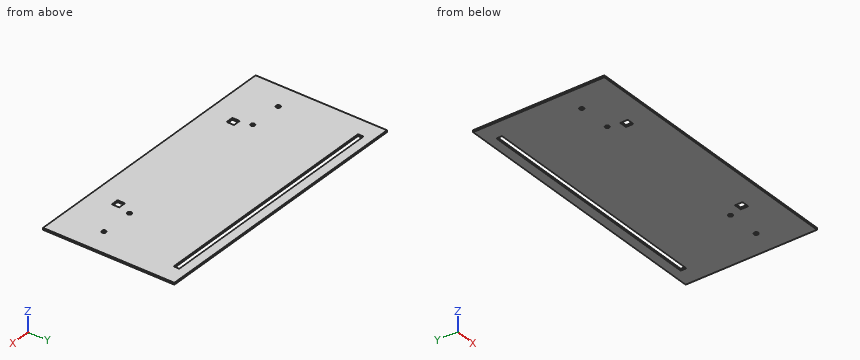
```python
from build123d import *

# Parameters (mm, degrees)
SK_PANEL_W            = 300
SK_PANEL_H            = 141.5
EX_PANEL_DEPTH        = 2
SK_LIGHTSLOT_W        = 260
SK_LIGHTSLOT_H        = 6
CUT_LIGHTSLOT_DEPTH   = 2
SK_CLIFFBOLTS_R       = 2.25
CUT_CLIFFBOLTS_DEPTH  = 2
SK_CLIFFCABLES_W      = 8
SK_CLIFFCABLES_H      = 8
CUT_CLIFFCABLES_DEPTH = 2


with BuildPart() as part:
    # SK_Panel → EX_Panel (new body)
    with BuildSketch(Plane.XY):
        with Locations((0, 70.75)):
            Rectangle(SK_PANEL_W, SK_PANEL_H)
    extrude(amount=EX_PANEL_DEPTH)

    # SK_LightSlot → CUT_LightSlot (cut)
    with BuildSketch(Plane.XY):
        with Locations((0, 128.5)):
            Rectangle(SK_LIGHTSLOT_W, SK_LIGHTSLOT_H)
    extrude(amount=CUT_LIGHTSLOT_DEPTH, mode=Mode.SUBTRACT)

    # SK_CliffBolts → CUT_CliffBolts (cut)
    with BuildSketch(Plane.XY):
        with Locations((123, 45)):
            Circle(SK_CLIFFBOLTS_R)
        with Locations((87, 45)):
            Circle(SK_CLIFFBOLTS_R)
        with Locations((-123, 45)):
            Circle(SK_CLIFFBOLTS_R)
        with Locations((-87, 45)):
            Circle(SK_CLIFFBOLTS_R)
    extrude(amount=CUT_CLIFFBOLTS_DEPTH, mode=Mode.SUBTRACT)

    # SK_CliffCables → CUT_CliffCables (cut)
    with BuildSketch(Plane.XY):
        with Locations((81, 28.5)):
            Rectangle(SK_CLIFFCABLES_W, SK_CLIFFCABLES_H)
        with Locations((-81, 28.5)):
            Rectangle(SK_CLIFFCABLES_W, SK_CLIFFCABLES_H)
    extrude(amount=CUT_CLIFFCABLES_DEPTH, mode=Mode.SUBTRACT)


solid = part.part
```
For this review, take the finished solid that the model builds, in its own axes (mm). Give positions to 0.01 mm unless a question says otherwise; leave off trailing zeros. Loops run counter-clockwise (first coordinate to the right, second up) from the corner with the lowest first, then second, coordinate; pieces in that order, holes last. Notation, with made-up numbers: M 66.25,20.5 L 81.25,20.5 A7 ccw 81.25,25.5 Z; hole C -18,50.5 d6. An arc over 180 degrees is marked long. One line per item, written item: value. Start each with the question number.
Q1. For L1, parallel to Y at x = -123, z = 0.7; L2, parallel to Y at x = 13, z = 1.15; L3, parallel to Y at x = 88, z = 0.3, list the stretches that pass through material, from the lowest coordinate up.
Q2. Add section A-A (x = -24). Give the boundary of the cut face in (y, z).
Q3. Clearance check with a flat-ended pin moving along its axis: pin 1 Ø1 at (x, z) = (4.5, 0.5) entering from -Y. State where the tip first meets the part, or that it passes through.
Q4. Add section B-B (z = 0.6). Give the boundary of the cut face in (x, y), and give its area (3 significant figures).
Reply:
1. L1: 0 to 42.75, 47.25 to 125.5, 131.5 to 141.5
1. L2: 0 to 125.5, 131.5 to 141.5
1. L3: 0 to 42.98, 47.02 to 125.5, 131.5 to 141.5
2. outline: M 0,0 L 125.5,0 L 125.5,2 L 0,2 Z; M 131.5,0 L 141.5,0 L 141.5,2 L 131.5,2 Z
3. pin 1: y = 0
4. outline: M -150,0 L 150,0 L 150,141.5 L -150,141.5 Z; hole M -130,125.5 L 130,125.5 L 130,131.5 L -130,131.5 Z; hole C -123,45 d4.5; hole C -87,45 d4.5; hole M -85,24.5 L -77,24.5 L -77,32.5 L -85,32.5 Z; hole M 77,24.5 L 85,24.5 L 85,32.5 L 77,32.5 Z; hole C 87,45 d4.5; hole C 123,45 d4.5
4. area: 40,700 mm²
